For this review, take the finished solid that the model builds, in its own axes (mm). A direction names the side the tool comes from. Give positions to 0.01 mm unless a question says otherwise; leave off trailing zeros. Order: outer loops, then holes, each group sorted by start corner. A loop starts at its lowest first (then second) coordinate and runs counter-clockwise, first axis right, second up.
from build123d import *

# Parameters (mm, degrees)
F2_W     = 25
F2_H     = 100
F2_R     = 7.5
F0_DEPTH = 15
F1_DEPTH = 25


with BuildPart() as f0:
    # F2 (on Top) → F0 (new body)
    with BuildSketch(Plane.XY):
        Rectangle(F2_W, F2_H)
        with Locations((0, 25)):
            Circle(F2_R, mode=Mode.SUBTRACT)
    extrude(amount=F0_DEPTH)

    # F3 (on face) → F1 (cut, through all)
    with BuildSketch(Plane(origin=(-12.5, 0, 0), x_dir=(0, -1, 0), z_dir=(-1, 0, 0))):
        with BuildLine():
            Line((8.109305, 5), (19.336069, 5))
            Line((19.336069, 5), (19.336069, 10))
            Line((19.336069, 10), (8.109305, 10))
            ThreePointArc((8.109305, 10), (5.609305, 7.5), (8.109305, 5))
        make_face()
    extrude(amount=-F1_DEPTH, mode=Mode.SUBTRACT)


solid = f0.part
1) We need section A-A on x = 0. Give the boundary of the cut face in (y, z).
Answer sheet:
outline: (-50, 0) - (17.5, 0) - (17.5, 15) - (-50, 15) - close; (32.5, 0) - (50, 0) - (50, 15) - (32.5, 15) - close; hole (-19.34, 5) - (-8.11, 5) arc R2.5 ccw to (-8.11, 10) - (-19.34, 10) - close
2) Draft analysis for pull direction Y (two halves, no side actions). For faces 3 (the face through (0, 50, 7)), 4 (the face through (0, -19.336, 7)), 5 (the face through (0, -50, 7)), state which applies: +Y half, -Y half, draft (parallel to the pull), parting line (faces both ways), or undercut.
Answer sheet:
face 3: +Y half
face 4: undercut
face 5: -Y half
3) Tool access review of faces 1 (the face through (0, 1, 0)), 2 (the face through (-0.18, -5.61, 7.55)): name each direction out of +Z, -Z, +X, -X, +Y, -Y from which nothing blocks a thin tool from reaching the whole face with its end or side.
Answer sheet:
face 1: -Z, +X, -X, +Y, -Y
face 2: +X, -X
4) We need section C-C on y = 25. Give the boundary of the cut face in (x, z).
Answer sheet:
outline: (-12.5, 0) - (-7.5, 0) - (-7.5, 15) - (-12.5, 15) - close; (7.5, 0) - (12.5, 0) - (12.5, 15) - (7.5, 15) - close
5) We need section D-D on x = 8.5. Give the boundary of the cut face in (y, z).
Answer sheet:
outline: (-50, 0) - (50, 0) - (50, 15) - (-50, 15) - close; hole (-19.34, 5) - (-8.11, 5) arc R2.5 ccw to (-8.11, 10) - (-19.34, 10) - close
6) We need section B-B on z = 7.25. Give the boundary of the cut face in (x, y).
Answer sheet:
outline: (-12.5, -50) - (12.5, -50) - (12.5, -19.34) - (-12.5, -19.34) - close; (-12.5, -5.62) - (12.5, -5.62) - (12.5, 50) - (-12.5, 50) - close; hole circle Ø15 at (0, 25)
7) To check wall thickness, follow line 1 (Y direction, x = 0, z = 8.5); line 2 (Y direction, x = 0, z = 9); line 3 (Y direction, x = 0, z = 3.5). State the ranges of each line that lie inside material, in increasing order.
Answer sheet:
line 1: y = -50 to -19.34, -5.82 to 17.5, 32.5 to 50
line 2: y = -50 to -19.34, -6.11 to 17.5, 32.5 to 50
line 3: y = -50 to 17.5, 32.5 to 50
